Check sheet for the modelled part. Datum: model origin and axes. Units: mm. Coordinates: 2 decimals unless noted, no trailing zeros. Loops run counter-clockwise (first coordinate to the right, second up) from the corner with the lowest first, then second, coordinate; pieces in that order, holes last. Notation, with made-up numbers: M 26,65.5 L 54,65.5 A27 ccw 54,88.5 Z; hole C -37.5,36 d9. An arc over 180 degrees is marked long. Answer as CSV lines item,"result". Start each with the question number.
from build123d import *

# Parameters (mm, degrees)
F1_DEPTH = 127
F2_R     = 12.7


with BuildPart() as f1:
    # F0 (on Top) → F1 (new body)
    with BuildSketch(Plane.XY):
        Polygon((-23.028424, 34.230471), (-23.028424, 61.040085), (-56.443118, 64.188562), (-56.443118, 34.230471), align=None)
    extrude(amount=F1_DEPTH)

    # F2
    f2_edges = [f1.edges().sort_by_distance(p)[0] for p in [
        (-39.735771, 62.614324, 127),
    ]]
    fillet(f2_edges, radius=F2_R)


solid = f1.part
Item 1: Sectioned sample at A-A, the plane z = 91.5. Record the boundary of the cut face in (x, y).
Item 2: Go/stop test with flat-tipped pins: pin 1 (1.5 mm diameter, centred on x = -47.5, z = 110, fed in from +Y); pin 2 (6 mm diameter, centred on x = -40, y = 61, fed in from +Z). Record where each tip stops, or that it passes through.
Item 3: Material ranges on line 1 (Z direction, x = -34.5, y = 50); line 2 (Z direction, x = -25, y = 54); line 3 (Y direction, x = -40.5, z = 8.5), recorded low to high. Write a range as from..to.
Reply:
1,outline,"M -56.44,34.23 L -23.03,34.23 L -23.03,61.04 L -56.44,64.19 Z"
2,pin 1,"y = 63.42"
2,pin 2,"z = 124.11"
3,line 1,"0..126.98"
3,line 2,"0..125.74"
3,line 3,"34.23..62.69"
